Could you check a few things on this model? Use its own coordinates, in mm. A direction names the side the tool comes from. Give positions to 0.01 mm unless a question says otherwise; leave off trailing zeros. Order: outer loops, then holes, each group sorted by start corner. A loop starts at its lowest first (then second) coordinate and runs counter-clockwise, first axis right, second up.
Autodesk Inventor part; units mm, degrees
ref_plane "Work Plane1" through (0, 27.7, 0) normal (0, 1, 0) x (1, 0, 0)
ref_plane "YZ Plane" through (0, 0, 0) normal (1, 0, 0) x (0, 1, 0)
ref_plane "XZ Plane" through (0, 0, 0) normal (0, 1, 0) x (-1, 0, 0)
sketch "Sketch1" plane through (0, 0, 0) normal (0, 1, 0) x (-1, 0, 0)
  line L0 (-10, 20) -> (10, 20)
  line L1 (10, 20) -> (10, -20)
  line L2 (10, -20) -> (-10, -20)
  line L3 (-10, -20) -> (-10, 20)
  line L4 (-10, 20) -> (10, -20) construction
  line L5 (10, 20) -> (-10, -20) construction
  point P0 (0, 0)
  dimension "d0" = 20
  dimension "d1" = 40
extrude "Extrusion1" add sketch "Sketch1" along normal blind 27.7
ref_plane "Work Plane1" through (0, 27.7, 0) normal (0, 1, 0) x (1, 0, 0)
sketch "Sketch2" plane through (0, 27.7, 0) normal (0, 1, 0) x (1, 0, 0)
  line L0 (-10, 20) -> (-10, -20)
  line L1 (-10, -20) -> (10, -20)
  line L2 (10, -20) -> (10, 20)
  line L3 (10, 20) -> (-10, 20)
  point P0 (0, 0)
extrude "Extrusion2" add sketch "Sketch2" along normal blind 12.7
sketch "Sketch3" plane through (0, 27.7, 0) normal (0, 1, 0) x (1, 0, 0)
  line L0 (10, -20) -> (10, 20)
  line L1 (10, 20) -> (-10, 20)
  line L2 (-10, 20) -> (-10, -20)
  line L3 (-10, -20) -> (10, -20)
  line L4 (10, -20) -> (-10, -20)
  line L5 (-10, -20) -> (-10, -27.25)
  line L6 (-10, -27.25) -> (10, -27.25)
  line L7 (10, -27.25) -> (10, -20)
  line L8 (10, 20) -> (-10, 20)
  line L9 (-10, 20) -> (-10, 27.25)
  line L10 (-10, 27.25) -> (10, 27.25)
  line L11 (10, 27.25) -> (10, 20)
  circle A0 centre (-5, -24.75) radius 2.25
  line L12 (-14, 0) -> (14, 0)
  line L13 (0, 38.15) -> (0, -38.15)
  circle A1 centre (-5, 24.75) radius 2.25
  circle A2 centre (5, -24.75) radius 2.25
  circle A3 centre (5, 24.75) radius 2.25
  line L14 (-6.25, -27.25) -> (-6.25, -26.6208)
  line L15 (-5, -27.25) -> (-5, -27)
  line L16 (-3.75, -27.25) -> (-3.75, -26.6208)
  line L17 (-6.25, 27.25) -> (-6.25, 26.6208)
  line L18 (-3.75, 27.25) -> (-3.75, 26.6208)
  line L19 (6.25, -27.25) -> (6.25, -26.6208)
  line L20 (3.75, -27.25) -> (3.75, -26.6208)
  line L21 (6.25, 27.25) -> (6.25, 26.6208)
  line L22 (3.75, 27.25) -> (3.75, 26.6208)
  point P0 (0, 0)
  point P1 (5.7141, 27.25)
  point P2 (4.2859, 27.25)
  point P3 (-4.2859, 27.25)
  point P4 (-5.7141, 27.25)
  point P5 (-5.7141, -27.25)
  point P6 (-4.2859, -27.25)
  point P7 (4.2859, -27.25)
  point P8 (5.7141, -27.25)
  point P9 (3.75, -26.6208)
  point P10 (6.25, 26.6208)
  point P11 (-6.25, 26.6208)
  dimension "d7" = 54.5
  dimension "d8" = 10
  dimension "d9" = 49.5
  dimension "d10" = 4.5
  dimension "d13" = 2.5
extrude "Extrusion3" add sketch "Sketch3" along normal blind 2.7 contours L7 L6 L19 A2 L20 L13 L3 | L13 L6 L16 A0 L14 L5 L3 | L1 L13 L10 L22 A3 L21 L11 | L1 L9 L10 L17 A1 L18 L13
sketch "Sketch4" plane through (0, 30.4, 0) normal (0, 1, 0) x (1, 0, 0)
  line L0 (-10, -20) -> (10, -20)
  line L1 (1, -24) -> (-1, -24)
  line L2 (-1, -24) -> (-1, -20)
  line L3 (-1, -20) -> (1, -20)
  line L4 (1, -20) -> (1, -24)
  line L5 (1, -24) -> (-1, -20) construction
  line L6 (-1, -24) -> (1, -20) construction
  line L7 (0, 38.15) -> (0, -38.15)
  line L8 (-14, 0) -> (14, 0)
  line L9 (1, 24) -> (-1, 24)
  line L10 (-1, 24) -> (-1, 20)
  line L11 (1, 20) -> (1, 24)
  line L12 (-1, 20) -> (1, 20)
  line L13 (10, 20) -> (-10, 20)
  point P0 (0, 0)
  point P1 (0, -22)
  point P2 (0, -22)
  point P3 (1, -20)
  dimension "d14" = 2
  dimension "d15" = 4
extrude "Extrusion4" add sketch "Sketch4" along normal blind 2
sketch "Sketch5" plane through (0, 40.4, 0) normal (0, 1, 0) x (1, 0, 0)
  circle A0 centre (0, 10) radius 3
  line L0 (10, -20) -> (10, 20)
  line L1 (10, 20) -> (-10, 20)
  line L2 (-10, 20) -> (-10, -20)
  line L3 (-10, -20) -> (10, -20)
  point P0 (0, 0)
  dimension "d18" = 6
  dimension "d19" = 30
extrude "Extrusion5" add sketch "Sketch5" along normal blind 5.6 contours A0
sketch "Sketch6" plane through (0, 46, -10) normal (0, 1, 0) x (1, 0, 0)
  circle A0 centre (0, 0) radius 3
  circle A1 centre (0, 0) radius 1.5
  point P0 (0, -10)
  dimension "d22" = 3
extrude "Extrusion6" cut sketch "Sketch6" against normal up to surface (5.6 mm away) contours A1
sketch "Sketch7" plane through (10, 0, -20) normal (0, 0, -1) x (-1, 0, 0)
  line L0 (6.8, 8) -> (13.2, 8)
  line L1 (13.2, 8) -> (13.2, 4)
  line L2 (13.2, 4) -> (6.8, 4)
  line L3 (6.8, 4) -> (6.8, 8)
  line L4 (6.8, 8) -> (13.2, 4) construction
  line L5 (13.2, 8) -> (6.8, 4) construction
  line L6 (0, 0) -> (20, 0)
  line L7 (10, 0) -> (10, 6)
  dimension "d25" = 6.4
  dimension "d26" = 4
  dimension "d27" = 8
extrude "Extrusion7" add sketch "Sketch7" along normal blind 6
properties part number "Servo"
Item 1: Imagine slicing it at B-B on x = 8.5. List the corners of the cut face in (y, z) for me.
Findings:
outline: (0, -20) - (27.7, -20) - (27.7, -27.25) - (30.4, -27.25) - (30.4, -20) - (40.4, -20) - (40.4, 20) - (30.4, 20) - (30.4, 27.25) - (27.7, 27.25) - (27.7, 20) - (0, 20) - close
Item 2: Imagine slicing it at A-A on z = 24.75. List the corners of the cut face in (x, y) for me, then the cut area to 3 significant figures.
Findings:
outline: (-10, 27.7) - (-7.25, 27.7) - (-7.25, 30.4) - (-10, 30.4) - close; (-2.75, 27.7) - (2.75, 27.7) - (2.75, 30.4) - (-2.75, 30.4) - close; (7.25, 27.7) - (10, 27.7) - (10, 30.4) - (7.25, 30.4) - close
area: 29.7 mm2
Item 3: Imagine slicing it at D-D on y = 38.5. List the corners of the cut face in (x, z) for me, then the cut area to 3 significant figures.
Findings:
outline: (-10, -20) - (10, -20) - (10, 20) - (-10, 20) - close
area: 800 mm2
Item 4: We'd pull the mould along X, two halves only. Please class faces 1 (the flat face through (3.2, 6, -23)), 2 (the flat face through (-0.1, 30.4, -24.5)), 3 (the cylindrical face through (4.92, 29.03, 22.5)): +X half, -X half, draft (parallel to the pull), parting line (faces both ways), or undercut.
Findings:
face 1: +X half
face 2: draft
face 3: undercut
Item 5: Please list where these lines run through material, in increasing order: line 1 along X through (y, z) = (28.45, 24.75); line 2 along X through (y, z) = (44, -10); line 3 along Z through (x, y) = (3.75, 4.5).
Findings:
line 1: x = -10 to -7.25, -2.75 to 2.75, 7.25 to 10
line 2: x = -3 to -1.5, 1.5 to 3
line 3: z = -20 to 20
Item 6: Imagine slicing it at C-C on x = 0. List the corners of the cut face in (y, z) for me, then the cut area to 3 significant figures.
Findings:
outline: (0, -20) - (4, -20) - (4, -26) - (8, -26) - (8, -20) - (27.7, -20) - (27.7, -27.25) - (30.4, -27.25) - (30.4, -24) - (32.4, -24) - (32.4, -20) - (40.4, -20) - (40.4, -13) - (46, -13) - (46, -11.5) - (40.4, -11.5) - (40.4, -8.5) - (46, -8.5) - (46, -7) - (40.4, -7) - (40.4, 20) - (32.4, 20) - (32.4, 24) - (30.4, 24) - (30.4, 27.25) - (27.7, 27.25) - (27.7, 20) - (0, 20) - close
area: 1,710 mm2
Item 7: For pin 1 (3 mm diameter, centred on x = -2.5, y = 35.5, fed in from +Z); pin 2 (4 mm diameter, centred on x = 8, y = 37.5, fed in from -Z); pin 3 (3.5 mm diameter, centred on x = 3.5, z = -22.5, fed in from +Y), each with a flat end and sliding along its axis, tell me the tip position at first contact or that it passes through.
Findings:
pin 1: stops at z = 20
pin 2: stops at z = -20
pin 3: stops at y = 30.4
Item 8: For faces 4 (the flat face through (0, 31, -24)), 5 (the cylindrical face through (0, 43, -7)), 6 (the flat face through (0, 32.4, 22)), 7 (the flat face through (1, 31, 22)), which set-ups out of +Z, -Z, +X, -X, +Y, -Y let a thin tool reach every point of the face, with its end or its side?
Findings:
face 4: -Z, +X, -X, +Y
face 5: +Y
face 6: +Z, +X, -X, +Y
face 7: +Z, +X, +Y
